Check sheet for the drawn part. Datum: minimum x, y, z corner. Units: mm. Coordinates: 2 decimals unless noted, no trailing zeros. Write each loop counter-clockwise with the first axis right and the second up, starting at its lowest first coordinate (ties: lowest second). Pieces come first, ordered by that corner, then holes. Notation, with made-up numbers: (-8.5, -2.5) -> (-1.5, -2.5) arc R19 ccw to (-1.5, 8.5) -> close; hole circle Ø8 at (-25, -10.75). An arc over 180 degrees is marked (long way). Answer in a Markdown table with one row per item. Add a question column.
1. Cross-section at A-A on y = 40. Record the cut outline in (x, z), and give its area (3 significant figures).
2. Mould release check, pull along X, two halves, no side actions. Record for the marked faces 1, 2, 3 and 4: pulls with the +X half, pulls with the -X half, needs draft (parallel to the pull), parting line crosses it, or undercut.
3. Cross-section at B-B on z = 2.75. Record the cut outline in (x, y), and give its area (3 significant figures).
4. Depth check by flat-ended pin: P1, Ø3, axis at x = 34, z = 6, coming from the +Y side. Enter the tip coordinate at first touch or a pass-through.
5. Cross-section at C-C on x = 5. Give the number of separate pieces and of enclosed holes in the cut face.
6. Cross-section at D-D on y = 8. Record the cut outline in (x, z).
7. Scan lines: L1, parallel to X at y = 39, z = 9.5; L2, parallel to X at y = 5, z = 7.75 (1 decimal); L3, parallel to Y at x = 33, z = 5.5 (1 decimal). Record each from-to range of solid material in increasing order. Write a range as from..to.
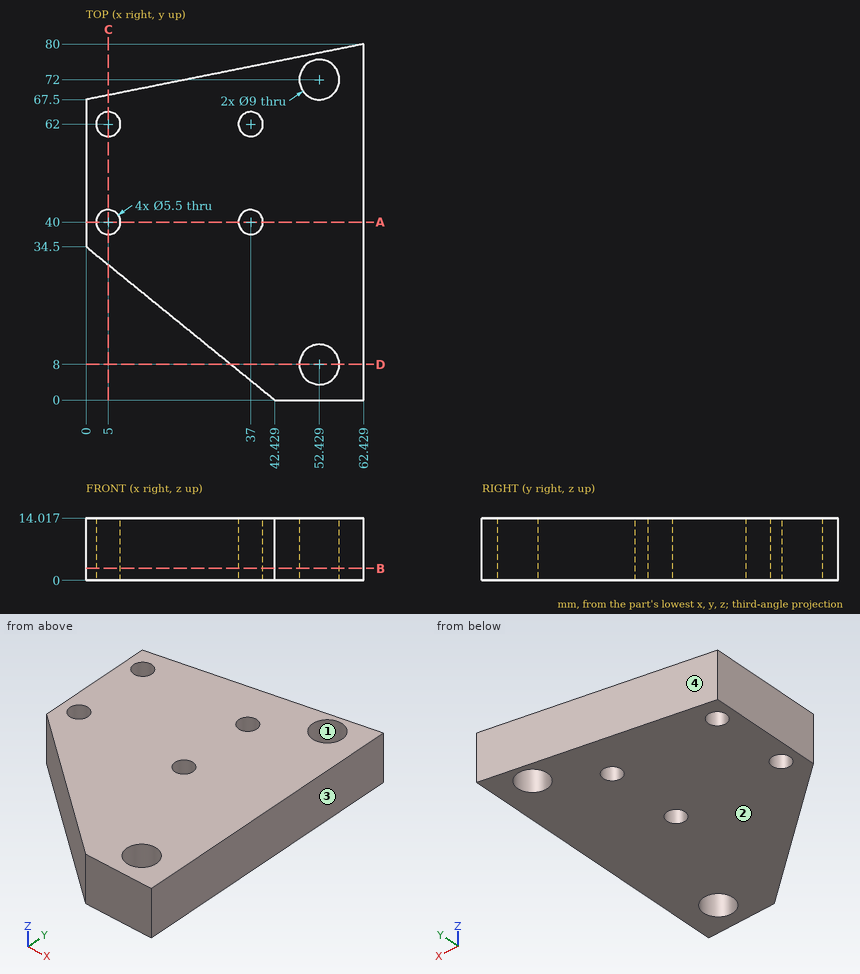
Results found:
| question | item | result |
|---|---|---|
| 1 | outline | (0, 0) -> (2.25, 0) -> (2.25, 14.02) -> (0, 14.02) -> close; (7.75, 0) -> (34.25, 0) -> (34.25, 14.02) -> (7.75, 14.02) -> close; (39.75, 0) -> (62.43, 0) -> (62.43, 14.02) -> (39.75, 14.02) -> close |
| 1 | area | 721 mm^2 |
| 2 | face 1 | undercut |
| 2 | face 2 | needs draft |
| 2 | face 3 | pulls with the +X half |
| 2 | face 4 | pulls with the -X half |
| 3 | outline | (0, 34.5) -> (42.43, 0) -> (62.43, 0) -> (62.43, 80) -> (0, 67.5) -> close; hole circle Ø5.5 at (5, 40); hole circle Ø5.5 at (5, 62); hole circle Ø5.5 at (37, 40); hole circle Ø5.5 at (37, 62); hole circle Ø9 at (52.43, 8); hole circle Ø9 at (52.43, 72) |
| 3 | area | 3,650 mm^2 |
| 4 | P1 | stops at y = 74.61 |
| 5 | separate pieces | 3 |
| 5 | enclosed holes | 0 |
| 6 | outline | (32.59, 0) -> (47.93, 0) -> (47.93, 14.02) -> (32.59, 14.02) -> close; (56.93, 0) -> (62.43, 0) -> (62.43, 14.02) -> (56.93, 14.02) -> close |
| 7 | L1 | x = 0..2.44, 7.56..34.44, 39.56..62.43 |
| 7 | L2 | x = 36.3..49.1, 55.8..62.4 |
| 7 | L3 | y = 7.7..74.1 |
